Answer from the drawing. Dimensions are ordinates in mm from the lowest x, y and z of the part. A direction names the side the tool comes from. Coordinates: 2 decimals unless noted, no trailing zeros. Write each loop counter-clockwise with the first axis right and the second up, starting at its lowest first coordinate (ties: lowest second). Pieces come first, ordered by that corner, then holes. Notation, with made-up numbers: (30, -27.75) - (38, -27.75) arc R27 cw to (38, 3.25) - close; hole circle Ø1 at (62, 32). An arc over 180 degrees is marked (long way). Return JSON: item names as keys, results as strings.
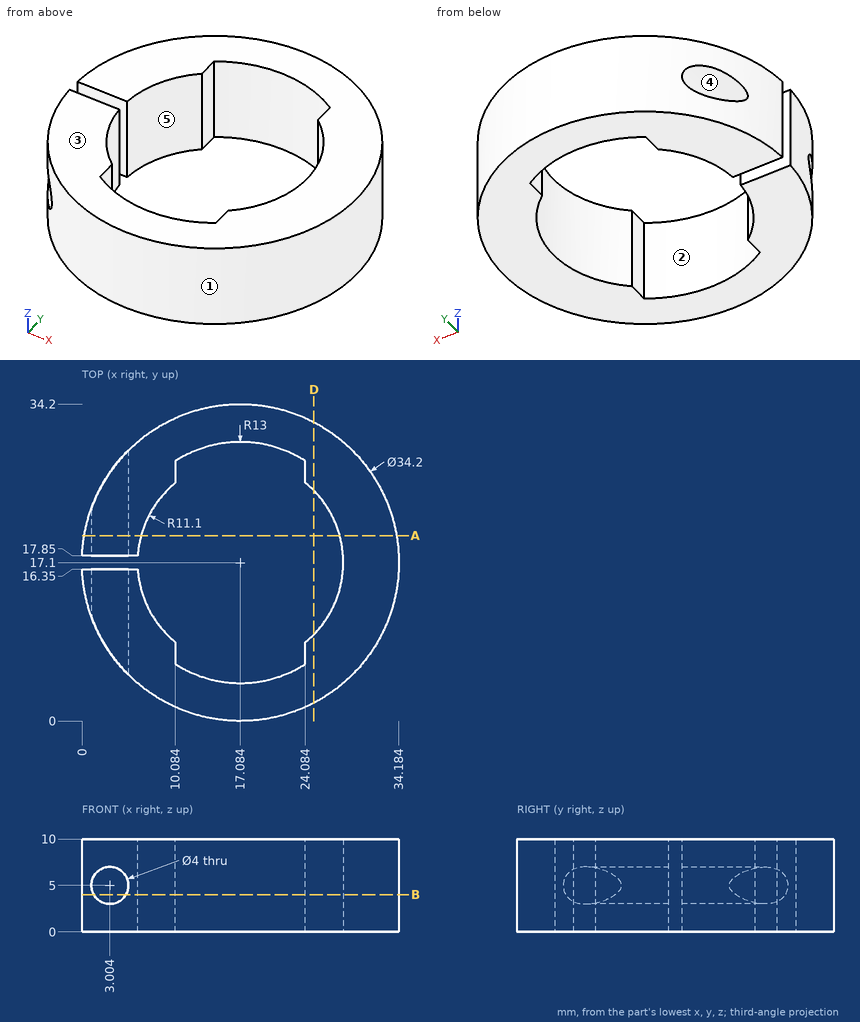
(1) Straight lines are drawn through the part: line 1 (X direction, y = 18, z = 5) (1 decimal); line 2 (X direction, y = 21, z = 5) (1 decimal); line 3 (Y direction, x = 5, z = 5.75). For each, find the intervals that lie inside material, in ascending order. Write a range as from..to.
Answer:
{"line 1": "0..1, 5..6, 28.1..34.2", "line 2": "0.4..1, 5..6.7, 27.5..33.7", "line 3": "5..16.35, 17.85..29.2"}
(2) Determine the mould class of the marked faces 1, 2 and 3 for opening direction Y: +Y half, -Y half, draft (parallel to the pull), parting line (faces both ways), or undercut.
Answer:
{"face 1": "parting line", "face 2": "undercut", "face 3": "draft"}
(3) A cutting plane is placed at A-A (y = 20). Determine the outline of the cut face in (x, z) (1 decimal).
Answer:
{"outline": "(0.2, 0) - (6.4, 0) - (6.4, 10) - (0.2, 10) - close; (27.8, 0) - (33.9, 0) - (33.9, 10) - (27.8, 10) - close; hole circle Ø4 at (3, 5)"}
(4) Flat-ended cylindrical pins translate along their axes: P1, Ø1.2, axis at y = 7.5, z = 7, coming from the +X side; P2, Ø1.2, axis at y = 26.5, z = 3, coming from the -X side; P3, Ø5, axis at x = 2.5, z = 3, coming from the +Y side. Find the tip coordinate at first contact, or state that the pin passes through.
Answer:
{"P1": "x = 31.62", "P2": "x = 2.42", "P3": "y = 29.2"}
(5) A cutting plane is placed at D-D (x = 25). Determine the outline of the cut face in (y, z).
Answer:
{"outline": "(1.94, 0) - (9.32, 0) - (9.32, 10) - (1.94, 10) - close; (24.88, 0) - (32.26, 0) - (32.26, 10) - (24.88, 10) - close"}
(6) A cutting plane is placed at B-B (z = 4). State how many separate pieces and enclosed holes the cut face has, and give its area (3 significant figures).
Answer:
{"separate pieces": "3", "enclosed holes": "0", "area": "405 mm²"}
(7) Which of the six approach directions +Z, -Z, +X, -X, +Y, -Y give full straight-line access (tool end or side, diameter ignored) to the marked faces 4 and 5?
Answer:
{"face 4": "+Y, -Y", "face 5": "+Z, -Z"}
